Part model, mm, in its own coordinate system. Face numbers are marked on the shaded views. A direction names the side the tool comes from. Round coordinates to 2 decimals unless told otherwise and drop trailing zeros. Write each loop counter-clockwise with the first axis right and the second up, starting at its lowest first coordinate (ties: lowest second). Pieces come first, ordered by that corner, then holes. Notation, with made-up numbers: M 40,0.5 L 70,0.5 A28 ccw 70,22.5 Z; hole C 12.25,3 d6. An arc over 180 degrees is marked long. Answer as a JSON object with one key per item and string values. Group by question number.
1. Which spindle directions (+Z, -Z, +X, -X, +Y, -Y) get a long thin tool onto all of the face, cutting with end or side? Do the marked faces 5, 6, 7 and 8. Say none if no direction does.
2. Band-saw the part on A-A, the plane z = -6. Write the cut outline in (x, y).
3. Drill centre lines: line 1 (Z direction, x = 6.25, y = 16); line 2 (Y direction, x = 7.75, z = 5); line 3 (Z direction, x = 5.5, y = 4). Where is each one in solid material? Low to high. Write a range as from..to.
4. Drop flat-ended pins along their axis: pin 1 (2.5 mm diameter, centred on x = 2, y = 0.5, fed in from -Z); pin 2 (3.5 mm diameter, centred on x = 1, y = 0.5, fed in from -Z); pin 3 (2 mm diameter, centred on x = 7, z = 36.5, fed in from +Y). Give the stop position or say it passes through.
5. Two-plate mould, pull along Z, no slides. Class the marked faces 1, 2, 3 and 4: +Z half, -Z half, draft (parallel to the pull), parting line (faces both ways), or undercut.
6. Band-saw the part on B-B, the plane x = 1. Count the separate pieces of the cut face and the enclosed holes in it, plus the area to 3 significant figures.
from build123d import *

# Parameters (mm, degrees)
SKETCH1_R           = 1.5
SKETCH1_W           = 12
SKETCH1_H           = 31
BOSS_EXTRUDE1_DEPTH = 8
FILLET1_R           = 6
FILLET2_R           = 15
FILLET3_R           = 5
SKETCH2_R           = 2
CUT_EXTRUDE1_DEPTH  = 50.689032995
BOSS_EXTRUDE2_START = 3
SKETCH3_R           = 4
SKETCH3_R_2         = 2
BOSS_EXTRUDE2_DEPTH = 3
CUT_EXTRUDE2_START  = -3
SKETCH4_W           = 16.5
SKETCH4_H           = 5
SKETCH4_R           = 1.5
CUT_EXTRUDE2_DEPTH  = 3


with BuildPart() as part:
    # Sketch1 → Boss-Extrude1 (new body)
    # profile 1 of 2: a face of its own
    with BuildSketch(Plane(origin=(0, 0, 0), x_dir=(0, 0, -1), z_dir=(1, 0, 0))):
        Polygon((-6, -5), (-6, -6), (38, -6), (38, 6), (26, 6), (-38, 6), (-38, -5), align=None)
        with Locations((24, 0)):
            Circle(SKETCH1_R, mode=Mode.SUBTRACT)
    # profile 2 of 2: a face of its own
    with BuildSketch(Plane(origin=(0, 0, 0), x_dir=(0, 0, -1), z_dir=(1, 0, 0))):
        with Locations((32, 21.5)):
            Rectangle(SKETCH1_W, SKETCH1_H)
        with Locations((32, 16)):
            Circle(SKETCH1_R, mode=Mode.SUBTRACT)
        with Locations((32, 32)):
            Circle(SKETCH1_R, mode=Mode.SUBTRACT)
    extrude(amount=BOSS_EXTRUDE1_DEPTH)

    # Fillet1
    fillet1_edges = [part.edges().sort_by_distance(p)[0] for p in [
        (4, 37, -26),
        (4, 37, -38),
    ]]
    fillet(fillet1_edges, radius=FILLET1_R - 0.0001)  # a hair under: the kernel refuses the full size

    # Fillet2
    fillet2_edges = [part.edges().sort_by_distance(p)[0] for p in [
        (4, -6, -38),
    ]]
    fillet(fillet2_edges, radius=FILLET2_R)

    # Fillet3
    fillet3_edges = [part.edges().sort_by_distance(p)[0] for p in [
        (4, 6, -26),
    ]]
    fillet(fillet3_edges, radius=FILLET3_R)

    # Sketch2 → Cut-Extrude1 (cut, through all)
    with BuildSketch(Plane(origin=(0, 6, 0), x_dir=(1, 0, 0), z_dir=(0, 1, 0))):
        with Locations(Location((4, -34, 0), (0, 0, 270))):
            Circle(SKETCH2_R)
        with Locations(Location((4, -10, 0), (0, 0, 270))):
            Circle(SKETCH2_R)
    extrude(amount=-CUT_EXTRUDE1_DEPTH, mode=Mode.SUBTRACT)

    # Sketch3 → Boss-Extrude2 (add)
    # profile 1 of 2: a face of its own
    with BuildSketch(Plane(origin=(0, 6, 0), x_dir=(1, 0, 0), z_dir=(0, 1, 0)).offset(BOSS_EXTRUDE2_START)):
        with Locations(Location((4, -10, 0), (0, 0, 180))):
            Circle(SKETCH3_R)
        with Locations(Location((4, -10, 0), (0, 0, 270))):
            Circle(SKETCH3_R_2, mode=Mode.SUBTRACT)
    # profile 2 of 2: a face of its own
    with BuildSketch(Plane(origin=(0, 6, 0), x_dir=(1, 0, 0), z_dir=(0, 1, 0)).offset(BOSS_EXTRUDE2_START)):
        with Locations(Location((4, -34, 0), (0, 0, 270))):
            Circle(SKETCH3_R)
        with Locations(Location((4, -34, 0), (0, 0, 270))):
            Circle(SKETCH3_R_2, mode=Mode.SUBTRACT)
    extrude(amount=-BOSS_EXTRUDE2_DEPTH)

    # Sketch4 → Cut-Extrude2 (cut)
    # profile 1 of 11: a face of its own
    with BuildSketch(Plane(origin=(8, 0, 0), x_dir=(0, 0, -1), z_dir=(1, 0, 0)).offset(CUT_EXTRUDE2_START)):
        with BuildLine():
            Line((-6.25, 3), (-6.25, -2))
            Line((-6.25, -2), (-3, -2))
            Line((-3, -2), (-3, -3))
            Line((-3, -3), (18.803847577, -3))
            ThreePointArc((18.803847577, -3), (18, 0), (18.803847577, 3))
            Line((18.803847577, 3), (-6.25, 3))
        make_face()
    # profile 2 of 11: a face of its own
    with BuildSketch(Plane(origin=(8, 0, 0), x_dir=(0, 0, -1), z_dir=(1, 0, 0)).offset(CUT_EXTRUDE2_START)):
        with Locations((-22, 0.5)):
            Rectangle(SKETCH4_W, SKETCH4_H)
    # profile 3 of 11: a face of its own
    with BuildSketch(Plane(origin=(8, 0, 0), x_dir=(0, 0, -1), z_dir=(1, 0, 0)).offset(CUT_EXTRUDE2_START)):
        with BuildLine():
            ThreePointArc((28.997628386, 10.805217551), (28.359995566, 7.86464272), (26.681204439, 5.367601211))
            ThreePointArc((26.681204439, 5.367601211), (29.103294359, 3.155374254), (30, 0))
            ThreePointArc((30, 0), (29.98714269, -0.392584271), (29.948625864, -0.783486015))
            ThreePointArc((29.948625864, -0.783486015), (33.662633595, 3.494707563), (35, 9))
            Line((35, 9), (35, 10.803847577))
            ThreePointArc((35, 10.803847577), (31.998630567, 10.000000156), (28.997628386, 10.805217551))
        make_face()
    # profile 4 of 11: a face of its own
    with BuildSketch(Plane(origin=(8, 0, 0), x_dir=(0, 0, -1), z_dir=(1, 0, 0)).offset(CUT_EXTRUDE2_START)):
        with BuildLine():
            Line((29, 26.803847577), (29, 21.196152423))
            ThreePointArc((29, 21.196152423), (32, 22), (35, 21.196152423))
            Line((35, 21.196152423), (35, 26.803847577))
            ThreePointArc((35, 26.803847577), (32, 26), (29, 26.803847577))
        make_face()
    # profile 5 of 11: a face of its own
    with BuildSketch(Plane(origin=(8, 0, 0), x_dir=(0, 0, -1), z_dir=(1, 0, 0)).offset(CUT_EXTRUDE2_START)):
        with BuildLine():
            Line((29, 31), (29, 30.197224362))
            ThreePointArc((29, 30.197224362), (32, 28.5), (35, 30.197224362))
            Line((35, 30.197224362), (35, 31))
            ThreePointArc((35, 31), (34.121320344, 33.121320344), (32, 34))
            ThreePointArc((32, 34), (29.878679656, 33.121320344), (29, 31))
        make_face()
        with Locations((32, 32)):
            Circle(SKETCH4_R, mode=Mode.SUBTRACT)
    # profile 6 of 11: a face of its own
    with BuildSketch(Plane(origin=(8, 0, 0), x_dir=(0, 0, -1), z_dir=(1, 0, 0)).offset(CUT_EXTRUDE2_START)):
        with BuildLine():
            ThreePointArc((35.5, 32), (31.064585653, 35.372684391), (29, 30.197224362))
            Line((29, 30.197224362), (29, 31))
            ThreePointArc((29, 31), (29.878679656, 33.121320344), (32, 34))
            ThreePointArc((32, 34), (34.121320344, 33.121320344), (35, 31))
            Line((35, 31), (35, 30.197224362))
            ThreePointArc((35, 30.197224362), (35.372684391, 31.064585653), (35.5, 32))
        make_face()
    # profile 7 of 11: a face of its own
    with BuildSketch(Plane(origin=(8, 0, 0), x_dir=(0, 0, -1), z_dir=(1, 0, 0)).offset(CUT_EXTRUDE2_START)):
        with BuildLine():
            ThreePointArc((35, 17.802775638), (32, 19.5), (29, 17.802775638))
            Line((29, 17.802775638), (29, 14.197224362))
            ThreePointArc((29, 14.197224362), (32, 12.5), (35, 14.197224362))
            Line((35, 14.197224362), (35, 17.802775638))
        make_face()
        with Locations((32, 16)):
            Circle(SKETCH4_R, mode=Mode.SUBTRACT)
    # profile 8 of 11: a face of its own
    with BuildSketch(Plane(origin=(8, 0, 0), x_dir=(0, 0, -1), z_dir=(1, 0, 0)).offset(CUT_EXTRUDE2_START)):
        with BuildLine():
            Line((35, 17.802775638), (35, 14.197224362))
            ThreePointArc((35, 14.197224362), (35.372684391, 15.064585653), (35.5, 16))
            ThreePointArc((35.5, 16), (35.372684391, 16.935414347), (35, 17.802775638))
        make_face()
    # profile 9 of 11: a face of its own
    with BuildSketch(Plane(origin=(8, 0, 0), x_dir=(0, 0, -1), z_dir=(1, 0, 0)).offset(CUT_EXTRUDE2_START)):
        with BuildLine():
            Line((29, 14.197224362), (29, 17.802775638))
            ThreePointArc((29, 17.802775638), (28.5, 16), (29, 14.197224362))
        make_face()
    # profile 10 of 11: a face of its own
    with BuildSketch(Plane(origin=(8, 0, 0), x_dir=(0, 0, -1), z_dir=(1, 0, 0)).offset(CUT_EXTRUDE2_START)):
        with BuildLine():
            ThreePointArc((23.761948832, 3.491895136), (23.104939246, 3.28188943), (22.432281937, 3.12925871))
            ThreePointArc((22.432281937, 3.12925871), (20.50257094, 0.134126691), (22.197224362, -3))
            Line((22.197224362, -3), (23, -3))
            ThreePointArc((23, -3), (24.748137439, -2.87198448), (26.458976757, -2.490669249))
            ThreePointArc((26.458976757, -2.490669249), (27.229273808, -1.349737262), (27.5, 0))
            ThreePointArc((27.5, 0), (26.389228004, 2.557653132), (23.761948832, 3.491895136))
        make_face()
        with Locations((24, 0)):
            Circle(SKETCH4_R, mode=Mode.SUBTRACT)
    # profile 11 of 11: a face of its own
    with BuildSketch(Plane(origin=(8, 0, 0), x_dir=(0, 0, -1), z_dir=(1, 0, 0)).offset(CUT_EXTRUDE2_START)):
        with BuildLine():
            Line((23, -3), (22.197224362, -3))
            ThreePointArc((22.197224362, -3), (24.415336527, -3.475269136), (26.458976757, -2.490669249))
            ThreePointArc((26.458976757, -2.490669249), (24.748137439, -2.87198448), (23, -3))
        make_face()
    cut_extrude2 = extrude(amount=CUT_EXTRUDE2_DEPTH, mode=Mode.SUBTRACT)

    # Mirror1: Cut-Extrude2 across plane
    add(cut_extrude2.mirror(Plane.ZY.offset(-4)), mode=Mode.SUBTRACT)


solid = part.part
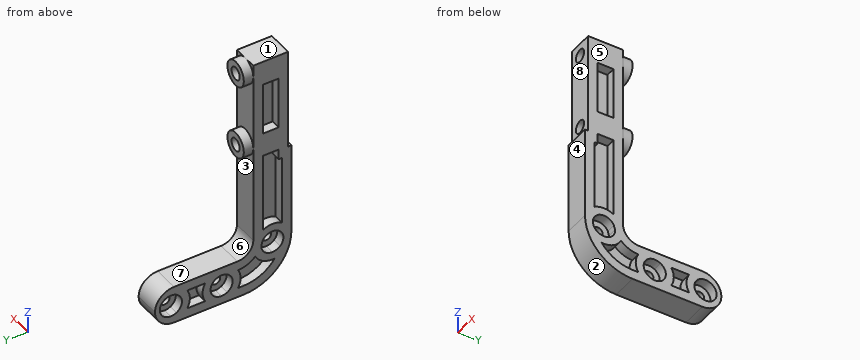
Worked answers:
{
 "1": {"face 5": "+Z, -Z, +X, +Y, -Y", "face 6": "+X, -X, +Y", "face 7": "+Z, +X, -X, +Y", "face 8": "+Z, +X, -X, -Y"},
 "2": {"outline": "M 0,-6 L 8,-6 L 8,-3 L 5,-3 L 5,3 L 8,3 L 8,6 L 0,6 L 0,3 L 3,3 L 3,-3 L 0,-3 Z"},
 "3": {"line 1": "z = -38..-35.5, -28.5..-26", "line 2": "y = -6..-2, 3..6", "line 3": "z = -37.14..-33.91, -28.47..8.68, 11.32..32.68, 35.32..38"},
 "4": {"pin 1": "stops at z = -36.13", "pin 2": "stops at z = -36.4", "pin 3": "stops at y = 9"},
 "5": {"face 1": "+Z half", "face 2": "-Z half", "face 3": "undercut", "face 4": "draft"},
 "6": {"separate pieces": "1", "enclosed holes": "7", "area": "802 mm^2"}
}
